Read the model definition and answer for the solid it produces. Units are mm, in the model's axes. A direction names the side the tool comes from. Coordinates: 2 decimals unless noted, no trailing zeros. Loops run counter-clockwise (first coordinate to the right, second up) from the corner with the lowest first, then second, coordinate; pieces in that order, holes last. Notation, with made-up numbers: (34, -17.75) - (72, -17.75) arc R31 ccw to (72, 8.25) - close; hole circle Ø7 at (0, 17.5). An arc over 180 degrees is marked (long way). Use CSV: the item, a comma, the result in double quotes.
```python
from build123d import *

# Parameters (mm, degrees)
F0_W     = 10
F0_H     = 4
F1_DEPTH = 5
F2_W     = 9
F2_H     = 3
F3_DEPTH = 4
F4_R     = 1.5
F5_DEPTH = 1


with BuildPart() as f1:
    # F0 (on Top) → F1 (new body)
    with BuildSketch(Plane.XY):
        Rectangle(F0_W, F0_H)
    extrude(amount=F1_DEPTH)

    # F2 (on face) → F3 (cut)
    with BuildSketch(Plane(origin=(0, 0, 0), x_dir=(1, 0, 0), z_dir=(0, 0, -1))):
        Rectangle(F2_W, F2_H)
    extrude(amount=-F3_DEPTH, mode=Mode.SUBTRACT)

    # F4 (on face) → F5 (join)
    with BuildSketch(Plane.XY.offset(5)):
        with Locations((-3, 0)):
            Circle(F4_R)
        with Locations((3, 0)):
            Circle(F4_R)
    extrude(amount=F5_DEPTH)


solid = f1.part
```
Q1. The part is cut by section C-C on y = 0. Determine the outline of the cut face in (x, z), and give its area (3 significant figures).
Reported:
outline,"(-5, 0) - (-4.5, 0) - (-4.5, 4) - (4.5, 4) - (4.5, 0) - (5, 0) - (5, 5) - (4.5, 5) - (4.5, 6) - (1.5, 6) - (1.5, 5) - (-1.5, 5) - (-1.5, 6) - (-4.5, 6) - (-4.5, 5) - (-5, 5) - close"
area,"20.0 mm²"
Q2. The part is cut by section D-D on x = 3. Determine the outline of the cut face in (y, z), and give its area (3 significant figures).
Reported:
outline,"(-2, 0) - (-1.5, 0) - (-1.5, 4) - (1.5, 4) - (1.5, 0) - (2, 0) - (2, 5) - (1.5, 5) - (1.5, 6) - (-1.5, 6) - (-1.5, 5) - (-2, 5) - close"
area,"11.0 mm²"
Q3. The part is cut by section A-A on z = 3.45. Determine the outline of the cut face in (x, y), and give its area (3 significant figures).
Reported:
outline,"(-5, -2) - (5, -2) - (5, 2) - (-5, 2) - close; hole (-4.5, -1.5) - (4.5, -1.5) - (4.5, 1.5) - (-4.5, 1.5) - close"
area,"13.0 mm²"
Q4. For a pull along Y with two mould halves and no side action, classify faces 4 (the face through (0, -2, 2)), 5 (the face through (-4.5, 0, 2)), 6 (the face through (0, 2, 2)) as +Y half, -Y half, draft (parallel to the pull), parting line (faces both ways), or undercut.
Reported:
face 4,"-Y half"
face 5,"undercut"
face 6,"+Y half"
Q5. The part is cut by section B-B on x = -1. Determine the outline of the cut face in (y, z), and give its area (3 significant figures).
Reported:
outline,"(-2, 0) - (-1.5, 0) - (-1.5, 4) - (1.5, 4) - (1.5, 0) - (2, 0) - (2, 5) - (-2, 5) - close"
area,"8.00 mm²"
Q6. A tool of negligible diameter and unlimited length cuts with its end or side. For faces 1 (the face through (5, 0, 2)), 2 (the face through (0, 1.5, 2)), 3 (the face through (0, 0, 5)), from which of +Z, -Z, +X, -X, +Y, -Y can it reach the whole face along a straight path? Write none if from no direction.
Reported:
face 1,"+Z, -Z, +X, +Y, -Y"
face 2,"-Z"
face 3,"+Z"
Q7. Find the intervals of material crossed by probe 1 along Y at (x, z) = (1, 1); probe 2 along X at (y, z) = (1.45, 3.95); probe 3 along Z at (x, y) = (-1, 1.3), in increasing order. Write a range as [from, to].
Reported:
probe 1,"y = [-2, -1.5], [1.5, 2]"
probe 2,"x = [-5, -4.5], [4.5, 5]"
probe 3,"z = [4, 5]"
Q8. Given P1, Ø1.5, axis at x = 0.5, y = -0.5, coming from the -Z side, flat-ended and moving along its own axis, determine where the tip first touches the part or whether it passes through.
Reported:
P1,"stops at z = 4"
